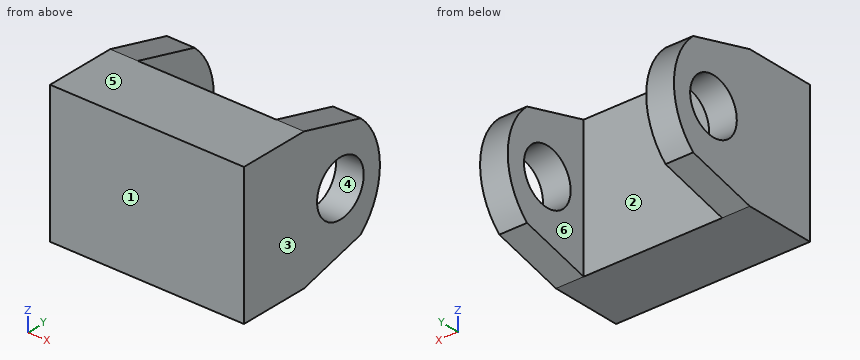
```python
from build123d import *

# Parameters (mm, degrees)
SKETCH1_W           = 35.56
SKETCH1_H           = 25.4
BOSS_EXTRUDE1_DEPTH = 13.0175
BOSS_EXTRUDE2_DEPTH = 5.08
SKETCH3_R           = 5.053169443
CUT_EXTRUDE1_DEPTH  = 36.56


with BuildPart() as part:
    # Sketch1 → Boss-Extrude1 (new body)
    with BuildSketch(Plane(origin=(0, 0, 0), x_dir=(1, 0, 0), z_dir=(0, 1, 0))):
        Rectangle(SKETCH1_W, SKETCH1_H)
    extrude(amount=BOSS_EXTRUDE1_DEPTH)

    # Sketch2 → Boss-Extrude2 (add)
    with BuildSketch(Plane(origin=(17.78, 0, 0), x_dir=(0, 0, -1), z_dir=(1, 0, 0))):
        with BuildLine():
            Line((-12.7, 13.0175), (-9.412998127, 25.284757994))
            ThreePointArc((-9.412998127, 25.284757994), (0, 29.45408338), (9.412998127, 25.284757994))
            Line((9.412998127, 25.284757994), (12.7, 13.0175))
            Line((12.7, 13.0175), (-12.7, 13.0175))
        make_face()
    boss_extrude2 = extrude(amount=-BOSS_EXTRUDE2_DEPTH)

    # Mirror1: Boss-Extrude2 across plane
    add(boss_extrude2.mirror(Plane(origin=(0, 0, 0), x_dir=(0, 0, 1), z_dir=(1, 0, 0))))

    # Sketch3 → Cut-Extrude1 (cut, through all)
    with BuildSketch(Plane(origin=(17.78, 0, 0), x_dir=(0, 0, -1), z_dir=(1, 0, 0))):
        with Locations((0, 20.8915)):
            Circle(SKETCH3_R)
    extrude(amount=-CUT_EXTRUDE1_DEPTH, mode=Mode.SUBTRACT)


solid = part.part
```
For this review, take the finished solid that the model builds, in its own axes (mm). Face numbers are marked on the shaded views. A direction names the side the tool comes from. Coordinates: 2 decimals unless noted, no trailing zeros. Write each loop counter-clockwise with the first axis right and the second up, starting at its lowest first coordinate (ties: lowest second). Pieces come first, ordered by that corner, then holes. Notation, with made-up numbers: (-20, 4) -> (12, 4) arc R31 cw to (12, 43) -> close; hole circle Ø9 at (14.25, -12). An arc over 180 degrees is marked (long way). Put each result on its own line as item: value.
Q1. The part is to be moulded in two halves that separate along Y. For the marked faces 1, 2, 3 and 4, say which applies: +Y half, -Y half, draft (parallel to the pull), parting line (faces both ways), or undercut.
From the geometry:
face 1: -Y half
face 2: +Y half
face 3: draft
face 4: undercut
Q2. Take a section at D-D, the plane z = -10.5. State the section outline as (x, y) points, then the cut area to 3 significant figures.
From the geometry:
outline: (-17.78, 0) -> (17.78, 0) -> (17.78, 21.23) -> (12.7, 21.23) -> (12.7, 13.02) -> (-12.7, 13.02) -> (-12.7, 21.23) -> (-17.78, 21.23) -> close
area: 546 mm2
Q3. Take a section at B-B, the plane y = 18.5. State the section outline as (x, z) points.
From the geometry:
outline: (-17.78, -11.23) -> (-12.7, -11.23) -> (-12.7, -4.45) -> (-17.78, -4.45) -> close; (-17.78, 4.45) -> (-12.7, 4.45) -> (-12.7, 11.23) -> (-17.78, 11.23) -> close; (12.7, -11.23) -> (17.78, -11.23) -> (17.78, -4.45) -> (12.7, -4.45) -> close; (12.7, 4.45) -> (17.78, 4.45) -> (17.78, 11.23) -> (12.7, 11.23) -> close
Q4. Tool access review of the marked faces 5 and 6: name each direction out of +Z, -Z, +X, -X, +Y, -Y from which nothing blocks a thin tool from reaching the whole face with its end or side.
From the geometry:
face 5: +Z, +X, -X, +Y, -Y
face 6: +Z, -Z, +Y
Q5. Take a section at C-C, the plane x = -15.5. State the section outline as (y, z) points.
From the geometry:
outline: (0, -12.7) -> (13.02, -12.7) -> (25.28, -9.41) arc R12.71 ccw to (25.28, 9.41) -> (13.02, 12.7) -> (0, 12.7) -> close; hole circle Ø10.11 at (20.89, 0)
Q6. Take a section at A-A, the plane z = 0. State the section outline as (x, y) points.
From the geometry:
outline: (-17.78, 0) -> (17.78, 0) -> (17.78, 15.84) -> (12.7, 15.84) -> (12.7, 13.02) -> (-12.7, 13.02) -> (-12.7, 15.84) -> (-17.78, 15.84) -> close; (-17.78, 25.94) -> (-12.7, 25.94) -> (-12.7, 29.45) -> (-17.78, 29.45) -> close; (12.7, 25.94) -> (17.78, 25.94) -> (17.78, 29.45) -> (12.7, 29.45) -> close
Q7. Clearance check with a flat-ended pin moving along its axis: pin 1 Ø8 at (x, z) = (-4.5, -5.5) entering from +Y. State where the tip first meets the part, or that it passes through.
From the geometry:
pin 1: stops at y = 13.02
Q8. Wall thickness on L1, parallel to Y at x = -16.4, z = 0; L2, parallel to X at y = 14, z = -4.25; L3, parallel to Y at x = -11.5, z = -5: over which ranges is each line inside the solid? List them lowest first.
From the geometry:
L1: y = 0 to 15.84, 25.94 to 29.45
L2: x = -17.78 to -12.7, 12.7 to 17.78
L3: y = 0 to 13.02
